```python
from build123d import *

# Parameters (mm, degrees)
SKETCH_1_W              = 280
SKETCH_1_H              = 284.25
SKETCH_1_W_2            = 216
SKETCH_1_H_2            = 220.25
EXTRUDE_1_DEPTH         = 3
FILLET_1_R              = 10
FILLET_2_R              = 5
HOLE_WIZARD_8_4_8_4_1_D = 8.4


with BuildPart() as part:
    # 草图1 → 凸台-拉伸1 (new body)
    with BuildSketch(Plane.XY):
        Rectangle(SKETCH_1_W, SKETCH_1_H)
        Rectangle(SKETCH_1_W_2, SKETCH_1_H_2, mode=Mode.SUBTRACT)
    extrude(amount=EXTRUDE_1_DEPTH)

    # 圆角1
    fillet_1_edges = [part.edges().sort_by_distance(p)[0] for p in [
        (140, -142.125, 1.5),
        (-140, -142.125, 1.5),
        (-140, 142.125, 1.5),
        (140, 142.125, 1.5),
    ]]
    fillet(fillet_1_edges, radius=FILLET_1_R)

    # 圆角2
    fillet_2_edges = [part.edges().sort_by_distance(p)[0] for p in [
        (108, -110.125, 1.5),
        (108, 110.125, 1.5),
        (-108, 110.125, 1.5),
        (-108, -110.125, 1.5),
    ]]
    fillet(fillet_2_edges, radius=FILLET_2_R)

    # Ø8.4 (8.4) 直径孔1 (through all)
    with Locations(Plane.XY.offset(3)):
        with Locations((120, -122.125), (-120, 122.125), (-120, -122.125), (120, 122.125)):
            Hole(HOLE_WIZARD_8_4_8_4_1_D / 2)


solid = part.part
```
The listing builds one solid part. Answer for the finished solid, in the listing's coordinates (mm). Coordinates: 2 decimals unless noted, no trailing zeros. Write each loop counter-clockwise with the first axis right and the second up, starting at its lowest first coordinate (ties: lowest second). Pieces come first, ordered by that corner, then holes. Notation, with made-up numbers: M 12,-1.5 L 16,-1.5 A8 cw 16,4.5 Z; hole C 56,-11 d6. An arc over 180 degrees is marked long. Use a Markdown table: item, result. Add a question column.
1. Section D-D (z = 0.7) is taken. Give the vertices of the cut face in (x, y) (3 decimals), plus the area to 3 significant figures.
2. Section B-B (y = -92.5) is taken. Give the vertices of the cut face in (x, z), plus the area to 3 significant figures.
3. Section C-C (x = -120) is taken. Give the vertices of the cut face in (y, z) (3 decimals), plus the area to 3 significant figures.
4. For a pull along X with two mould halves and no side action, classify faces 1 (the cylindrical face through (-123.88, 120.52, 1.48)), 2 (the cylindrical face through (136.993, -139.273, 1.521)), 3 (the cylindrical face through (-137.148, -139.118, 1.521)) as +X half, -X half, draft (parallel to the pull), parting line (faces both ways), or undercut.
5. Straight lines are drawn through the part: line 1 along Y through (x, z) = (-120, 2.45) (3 decimals); line 2 along X through (y, z) = (2, 1.7); line 3 along Y through (x, z) = (43, 0.35) (3 decimals). For each, find the intervals that lie inside material, in ascending order. Write a range as [from, to].
6. Section A-A (x = -64.5) is taken. Give the vertices of the cut face in (y, z) (3 decimals), plus the area to 3 significant figures.
7. Given P1, Ø6.5, axis at x = 120, y = 122.125, coming from the -Z side, flat-ended and moving along its own axis, determine where the tip first touches the part or whether it passes through.
Data:
| question | item | result |
|---|---|---|
| 1 | outline | M -140,-132.125 A10 ccw -130,-142.125 L 130,-142.125 A10 ccw 140,-132.125 L 140,132.125 A10 ccw 130,142.125 L -130,142.125 A10 ccw -140,132.125 Z; hole C -120,-122.125 d8.4; hole C -120,122.125 d8.4; hole M -108,-105.125 A5 ccw -103,-110.125 L 103,-110.125 A5 ccw 108,-105.125 L 108,105.125 A5 ccw 103,110.125 L -103,110.125 A5 ccw -108,105.125 Z; hole C 120,-122.125 d8.4; hole C 120,122.125 d8.4 |
| 1 | area | 31,700 mm2 |
| 2 | outline | M -140,0 L -108,0 L -108,3 L -140,3 Z; M 108,0 L 140,0 L 140,3 L 108,3 Z |
| 2 | area | 192 mm2 |
| 3 | outline | M -142.125,0 L -126.325,0 L -126.325,3 L -142.125,3 Z; M -117.925,0 L 117.925,0 L 117.925,3 L -117.925,3 Z; M 126.325,0 L 142.125,0 L 142.125,3 L 126.325,3 Z |
| 3 | area | 802 mm2 |
| 4 | face 1 | undercut |
| 4 | face 2 | +X half |
| 4 | face 3 | -X half |
| 5 | line 1 | y = [-142.125, -126.325], [-117.925, 117.925], [126.325, 142.125] |
| 5 | line 2 | x = [-140, -108], [108, 140] |
| 5 | line 3 | y = [-142.125, -110.125], [110.125, 142.125] |
| 6 | outline | M -142.125,0 L -110.125,0 L -110.125,3 L -142.125,3 Z; M 110.125,0 L 142.125,0 L 142.125,3 L 110.125,3 Z |
| 6 | area | 192 mm2 |
| 7 | P1 | passes through |
